Can you work these out from the model? Positions are in its coordinate system, mm. Give positions to 0.01 mm unless a question says otherwise; leave off trailing zeros. Order: outer loops, then holes, each group sorted by start corner. A loop starts at its lowest first (then second) coordinate and runs counter-clockwise, first axis right, second up. Notation, with made-up numbers: (38, -23) - (86, -23) arc R20 ccw to (86, -12) - close; hole circle Ø8 at (31.5, 39.25). An arc over 180 degrees is marked (long way). One line per question, with ' | ' between items.
```python
from build123d import *

# Parameters (mm, degrees)
F1_DEPTH = 3.175
F3_D     = 6.35


with BuildPart() as f1:
    # F0 (on Top) → F1 (new body)
    with BuildSketch(Plane.XY):
        with BuildLine():
            ThreePointArc((-9.552005, 9.498045), (-12.993834, -4.509148), (-1.121279, -12.7))
            Line((-1.121279, -12.7), (24.278721, -12.7))
            ThreePointArc((24.278721, -12.7), (33.258978, -8.980256), (36.978721, 0))
            Line((36.978721, 0), (36.978721, 50.8))
            Line((36.978721, 50.8), (-9.552005, 9.498045))
        make_face()
    extrude(amount=F1_DEPTH)

    # F3 (through all)
    with Locations(Plane.XY.offset(3.175)):
        with Locations((24.278721, 0), (-1.121279, 0)):
            Hole(F3_D / 2)


solid = f1.part
```
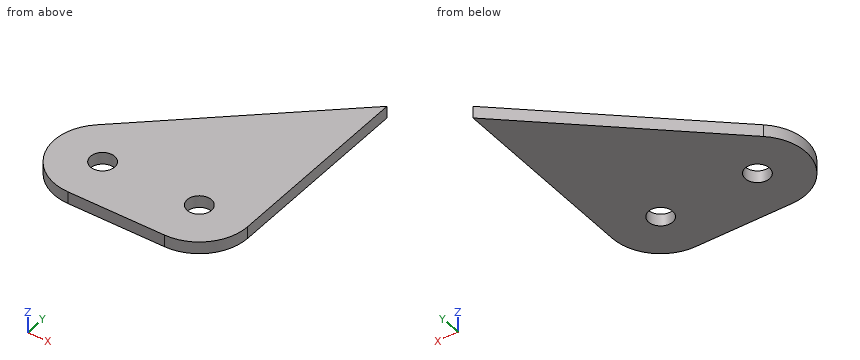
(1) If I drill on line 1 (Y direction, x = 26.5, z = 1.15); line 2 (Y direction, x = 24, z = 0.7); line 3 (Y direction, x = 17, z = 3), over which ranges is the centre line in solid material (lowest first)?
Answer below:
line 1: -12.5 to -2.27, 2.27 to 41.5 | line 2: -12.7 to -3.16, 3.16 to 39.28 | line 3: -12.7 to 33.07
(2) Imagine slicing it at B-B (x = 26). List the corners of the cut face in (y, z) for me (3 decimals).
Answer below:
outline: (-12.583, 0) - (-2.668, 0) - (-2.668, 3.175) - (-12.583, 3.175) - close; (2.668, 0) - (41.055, 0) - (41.055, 3.175) - (2.668, 3.175) - close
(3) Imagine slicing it at C-C (x = 0.5). List the corners of the cut face in (y, z) for me (3 decimals), and give its area (3 significant figures).
Answer below:
outline: (-12.7, 0) - (-2.73, 0) - (-2.73, 3.175) - (-12.7, 3.175) - close; (2.73, 0) - (18.42, 0) - (18.42, 3.175) - (2.73, 3.175) - close | area: 81.5 mm^2
(4) Imagine slicing it at A-A (z = 2.4). List the corners of the cut face in (x, y) for me (3 decimals), and give its area (3 significant figures).
Answer below:
outline: (-9.552, 9.498) arc R12.7 ccw to (-1.121, -12.7) - (24.279, -12.7) arc R12.7 ccw to (36.979, 0) - (36.979, 50.8) - close; hole circle Ø6.35 at (-1.121, 0); hole circle Ø6.35 at (24.279, 0) | area: 1,940 mm^2
(5) Imagine slicing it at D-D (y = 36.5). List the corners of the cut face in (x, z) for me (3 decimals), and give its area (3 significant figures).
Answer below:
outline: (20.868, 0) - (36.979, 0) - (36.979, 3.175) - (20.868, 3.175) - close | area: 51.2 mm^2
